from build123d import *

# Parameters (mm, degrees)
SKETCH1_R               = 22.5
BOSS_EXTRUDE1_DEPTH     = 15
BOSS_EXTRUDE2_DEPTH     = 22
CUT_EXTRUDE1_DEPTH      = 61
CUT_EXTRUDE1_DEPTH_BACK = 61
FILLET1_R               = 100
CUT_EXTRUDE2_START      = -27.5
CUT_EXTRUDE2_DEPTH      = 4
CUT_EXTRUDE2_TAPER      = 5
CUT_EXTRUDE3_DEPTH      = 61.0000001
CUT_EXTRUDE3_DEPTH_BACK = 61.0000001


with BuildPart() as part:
    # Sketch1 → Boss-Extrude1 (new body)
    with BuildSketch(Plane(origin=(0, 0, 0), x_dir=(0, 0, -1), z_dir=(1, 0, 0))):
        Circle(SKETCH1_R)
    extrude(amount=BOSS_EXTRUDE1_DEPTH)

    # Sketch2 → Boss-Extrude2 (add)
    with BuildSketch(Plane(origin=(15, 0, 0), x_dir=(0, 0, -1), z_dir=(1, 0, 0))):
        with BuildLine():
            Line((-27.5, 0), (-27.5, -20))
            Line((-27.5, -20), (-60, -40))
            ThreePointArc((-60, -40), (0, -100), (60, -40))
            Line((60, -40), (27.5, -20))
            Line((27.5, -20), (27.5, 0))
            ThreePointArc((27.5, 0), (0, 27.5), (-27.5, 0))
        make_face()
    extrude(amount=BOSS_EXTRUDE2_DEPTH)

    # Sketch3 → Cut-Extrude1 (cut, two sides)
    with BuildSketch(Plane.XY) as cut_extrude1_sk:
        Polygon((27, 27.5), (37, 27.5), (37, -62.5), align=None)
    extrude(amount=CUT_EXTRUDE1_DEPTH, mode=Mode.SUBTRACT)
    extrude(cut_extrude1_sk.sketch, amount=-CUT_EXTRUDE1_DEPTH_BACK, mode=Mode.SUBTRACT)

    # Fillet1
    fillet1_edges = [part.edges().sort_by_distance(p)[0] for p in [
        (37, -62.5, 0),
    ]]
    fillet(fillet1_edges, radius=FILLET1_R)

    # Sketch4 → Revolve1 (revolve)
    with BuildSketch(Plane.XY):
        Polygon((25.790103906, -17.5), (60, -17.5), (60, -25), (75, -25), (75, -27.5), (125, -27.5), (125, -40), (25.790103906, -40), align=None)
    revolve(axis=Axis((125, -40, 0), (-1, 0, 0)))

    # Sketch5 → Cut-Extrude2 (cut)
    with BuildSketch(Plane(origin=(0, 0, 0), x_dir=(1, 0, 0), z_dir=(0, 1, 0)).offset(CUT_EXTRUDE2_START)):
        with BuildLine():
            ThreePointArc((97, 4), (93, 0), (97, -4))
            Line((97, -4), (117, -4))
            ThreePointArc((117, -4), (121, 0), (117, 4))
            Line((117, 4), (97, 4))
        make_face()
    extrude(amount=-CUT_EXTRUDE2_DEPTH, taper=CUT_EXTRUDE2_TAPER, mode=Mode.SUBTRACT)

    # Mirror1: part across plane


with BuildPart() as part_1:
    add(part.part)
    add(part.part.mirror(Plane(origin=(0, 0, 0), x_dir=(0, 0, 1), z_dir=(1, 0, 0))))

    # Sketch6 → Cut-Extrude3 (cut, two sides)
    with BuildSketch(Plane.XY) as cut_extrude3_sk:
        Polygon((-75, -520.584014882), (-75, -67.635702331), (-75, -7.558349371), (-75, 445.38996318), (-980.896625102, 445.38996318), (-980.896625102, -520.584014882), align=None)
    extrude(amount=CUT_EXTRUDE3_DEPTH, mode=Mode.SUBTRACT)
    extrude(cut_extrude3_sk.sketch, amount=-CUT_EXTRUDE3_DEPTH_BACK, mode=Mode.SUBTRACT)


solid = part_1.part
Source: CAD feature listing. Evaluate the final solid. Frame: model axes, mm. A direction names the side the tool comes from. Round coordinates to 2 decimals unless told otherwise and drop trailing zeros. Loops run counter-clockwise (first coordinate to the right, second up) from the corner with the lowest first, then second, coordinate; pieces in that order, holes last. Notation, with made-up numbers: M 6.25,22.25 L 52.25,22.25 A30 cw 52.25,57.25 Z; hole C -3.75,62 d11. An arc over 180 degrees is marked long. Return JSON: item names as keys, results as strings. Group by question number.
1. Section query A-A on z = -42. Output: boundary loops of the cut face in (x, y), and give its area (3 significant figures).
2. Mould query, pull axis X, two halves, no side actions, for faces 1 (the face through (-24.61, -29.86, 43.52)), 2 (the face through (-37, -80, 1)), 3 (the face through (15, -50, 1)). Classes: released by +X, released by -X, zero draft, split by the parting line, or undercut.
3. Section query B-B on x = -19.5. Output: boundary loops of the cut face in (y, z), and give its area (3 significant figures).
4. Reachability of faces 4 (the face through (0.21, -19.961, -10.382)), 5 (the face through (-46.196, -19.216, 8.618)), 6 (the face through (46.196, -19.216, 8.618)), 7 (the face through (107, -31.5, 0)) from +Z, -Z, +X, -X, +Y, -Y: full face, straight path, thin tool, end or side. Return the list, or none.
5. Pin query (flat end, axial travel): pin 1 (16 mm diameter, centred on y = -83.5, z = -12.5, fed in from -X); pin 2 (19 mm diameter, centred on x = -20, y = -9, fed in from +Z); pin 3 (10 mm diameter, centred on x = -28, y = -16.5, fed in from +Z). Return the tip coordinate at first contact, or that it passes through.
6. Section query C-C on y = -37. Output: boundary loops of the cut face in (x, z) (3 decimals).
7. Material intervals for line 1 along X through (y, z) = (-71.5, -18); line 2 along X through (y, z) = (-57, 47.5); line 3 along Z through (x, y) = (29, -3), sorted ascending. Write a range as from..to.
Checks:
{
 "1": {"outline": "M -37,-82.85 L -15,-82.85 L -15,-28.92 L -33.27,-28.92 L -36.39,-57 A100 ccw -37,-68.04 Z; M 15,-82.85 L 37,-82.85 L 37,-68.04 A100 ccw 36.39,-57 L 33.27,-28.92 L 15,-28.92 Z", "area": "2,250 mm²"},
 "2": {"face 1": "zero draft", "face 2": "released by -X", "face 3": "undercut"},
 "3": {"outline": "M -40,-60 L -20,-27.5 L 0,-27.5 A27.5 ccw 0,27.5 L -20,27.5 L -40,60 A60 ccw Z", "area": "9,690 mm²"},
 "4": {"face 4": "none", "face 5": "-X", "face 6": "+X", "face 7": "+Y"},
 "5": {"pin 1": "stops at x = -37", "pin 2": "stops at z = 27.5", "pin 3": "stops at z = 29.94"},
 "6": {"outline": "M -75,-14.697 L -60,-14.697 L -60,-22.299 L -34.167,-22.299 L -34.167,-55.125 L -15,-55.125 L -15,55.125 L -34.167,55.125 L -34.167,22.299 L -60,22.299 L -60,14.697 L -75,14.697 Z; M 15,-55.125 L 34.167,-55.125 L 34.167,-22.299 L 60,-22.299 L 60,-14.697 L 75,-14.697 L 75,-12.135 L 125,-12.135 L 125,12.135 L 75,12.135 L 75,14.697 L 60,14.697 L 60,22.299 L 34.167,22.299 L 34.167,55.125 L 15,55.125 Z"},
 "7": {"line 1": "x = -37..-15, 15..37", "line 2": "x = -36.39..-15, 15..36.39", "line 3": "z = -27.5..27.5"}
}
